```python
from build123d import *

# Parameters (mm, degrees)
CROQUIS1_R              = 10
SALIENTE_EXTRUIR1_DEPTH = 3
CROQUIS2_R              = 0.75
CROQUIS4_R              = 7.5
SALIENTE_EXTRUIR2_DEPTH = 20
CROQUIS3_R              = 5
CORTAR_EXTRUIR1_DEPTH   = 28


with BuildPart() as part:
    # Croquis1 → Saliente-Extruir1 (new body)
    with BuildSketch(Plane(origin=(0, 0, 0), x_dir=(1, 0, 0), z_dir=(0, 1, 0))):
        with Locations(Location((0, 0, 0), (0, 0, 270))):
            Circle(CROQUIS1_R)
    extrude(amount=SALIENTE_EXTRUIR1_DEPTH)

    # Croquis2 → Cortar-Revolución1 (revolve, cut)
    with BuildSketch(Plane(origin=(0, 0, 0), x_dir=(0, 0, -1), z_dir=(1, 0, 0)), mode=Mode.PRIVATE) as cortar_revoluci_n1_sk:
        with Locations((10, 1.5)):
            Circle(CROQUIS2_R)
    revolve(cortar_revoluci_n1_sk.sketch.rotate(Axis((0, 3, 0), (0, -1, 0)), 180), axis=Axis((0, 3, 0), (0, -1, 0)), mode=Mode.SUBTRACT)

    # Croquis4 → Saliente-Extruir2 (add)
    with BuildSketch(Plane.XZ):
        with Locations(Location((0, 0, 0), (0, 0, 90))):
            Circle(CROQUIS4_R)
    extrude(amount=SALIENTE_EXTRUIR2_DEPTH)

    # Croquis3 → Cortar-Extruir1 (cut, through all)
    with BuildSketch(Plane(origin=(0, 3, 0), x_dir=(1, 0, 0), z_dir=(0, 1, 0))):
        with Locations(Location((0, 0, 0), (0, 0, 270))):
            Circle(CROQUIS3_R)
    extrude(amount=-CORTAR_EXTRUIR1_DEPTH, mode=Mode.SUBTRACT)


solid = part.part
```
Here's how the part is built. I have some questions about the finished solid (model axes, mm). A direction names the side the tool comes from. Coordinates: 2 decimals unless noted, no trailing zeros. Order: outer loops, then holes, each group sorted by start corner. A loop starts at its lowest first (then second) coordinate and runs counter-clockwise, first axis right, second up. Notation, with made-up numbers: M 29.5,-34 L 58.5,-34 A17 cw 58.5,-8 Z; hole C 45,79 d8. An arc over 180 degrees is marked long. Answer as a JSON object with one key per item and string values. Group by question number.
(1) Which directions (+Z, -Z, +X, -X, +Y, -Y) give clear straight access to the entire face, cutting with the end or side of a thin tool? Please do faces 1 (the face through (-9.76, 2.62, -2.17)), 2 (the face through (7, 0, 4)).
(2) Suppose I cut it at C-C, the plane y = -17. Please give me the cut outline in (x, z), then the cut area to 3 significant figures.
(3) For pin 1 (1.5 mm diameter, centred on x = -7, y = -6, fed in from +Z); pin 2 (2 mm diameter, centred on x = 3, y = 0.5, fed in from +Z); pin 3 (1 mm diameter, centred on x = 2.5, y = -12.5, fed in from -Z), each with a flat end and sliding along its axis, tell me the tip position at first contact or that it passes through.
(4) Suppose I cut it at A-A, the plane x = 0. Please give me the cut outline in (y, z), then the cut area to 3 significant figures.
(5) I need wall thicknesses on probe 1 along X at (y, z) = (-6.25, 0); probe 2 along Y at (x, z) = (-6, -5); probe 3 along Z at (x, y) = (4, -17). Which ranges of each line are inside material? Lowest first, please.
(6) Suppose I cut it at B-B, the plane z = 0. Please give me the cut outline in (x, y).
Values found:
{
 "1": {"face 1": "+Y, -Y", "face 2": "-Y"},
 "2": {"outline": "C 0,0 d15; hole C 0,0 d10", "area": "98.2 mm^2"},
 "3": {"pin 1": "stops at z = 4.15", "pin 2": "stops at z = 9.8", "pin 3": "stops at z = -7.23"},
 "4": {"outline": "M -20,-7.5 L 0,-7.5 L 0,-10 L 0.75,-10 A0.75 cw 2.25,-10 L 3,-10 L 3,-5 L -20,-5 Z; M -20,5 L 3,5 L 3,10 L 2.25,10 A0.75 cw 0.75,10 L 0,10 L 0,7.5 L -20,7.5 Z", "area": "128 mm^2"},
 "5": {"probe 1": "x = -7.5 to -5, 5 to 7.5", "probe 2": "y = 0 to 3", "probe 3": "z = -6.34 to -3, 3 to 6.34"},
 "6": {"outline": "M -10,0 L -7.5,0 L -7.5,-20 L -5,-20 L -5,3 L -10,3 L -10,2.25 A0.75 cw -10,0.75 Z; M 5,-20 L 7.5,-20 L 7.5,0 L 10,0 L 10,0.75 A0.75 cw 10,2.25 L 10,3 L 5,3 Z"}
}
